Here's the drawing with two shaded views (mm, measured from the low corner). I have some questions. A direction names the side the tool comes from. Coordinates: 2 decimals unless noted, no trailing zeros. Loops run counter-clockwise (first coordinate to the right, second up) from the corner with the lowest first, then second, coordinate; pieces in that order, holes last. Notation, with made-up numbers: (-8.75, 28) - (27.25, 28) arc R32 ccw to (27.25, 55) - close; hole circle Ø9 at (-14, -40). An arc over 180 degrees is marked (long way). One line per item, written item: value. Start each with the question number.
(1) If we mould it in two halves opening along Z, with no side actions, what happens to the marked faces 3, 4 and 5? For each: pulls with the +Z half, pulls with the -Z half, needs draft (parallel to the pull), parting line crosses it, or undercut.
(2) If we section it at A-A on y = 8: Write out the boundary of the cut face in (x, z) (3 decimals), then the cut area to 3 significant figures.
(3) If I drill on line 1 along Z through (x, y) = (2, 8) (3 decimals); line 2 along Z through (x, y) = (5.75, 8) (3 decimals), over which ranges is the centre line in solid material (lowest first)? Write a range as from..to.
(4) I'm going to push flat-ended pins straight in: P1, Ø3, axis at x = 8, y = 13.5, coming from the +Z side; P2, Ø4, axis at x = 5.5, y = 3, coming from the +Z side. Where does each tip first touch, or does it pass through?
(5) If we section it at C-C on x = 9.25: Write out the boundary of the cut face in (y, z) (3 decimals), then the cut area to 3 significant figures.
(6) On a 3-axis mill with a long thin cutter (end or side, diameter ignored), from which of +Z, -Z, +X, -X, +Y, -Y can I reach the whole of each face in a straight line? I mean the marked faces 1 and 2. Say none if no direction works.
(7) If we section it at B-B on x = 6.75: Write out the boundary of the cut face in (y, z) (3 decimals).
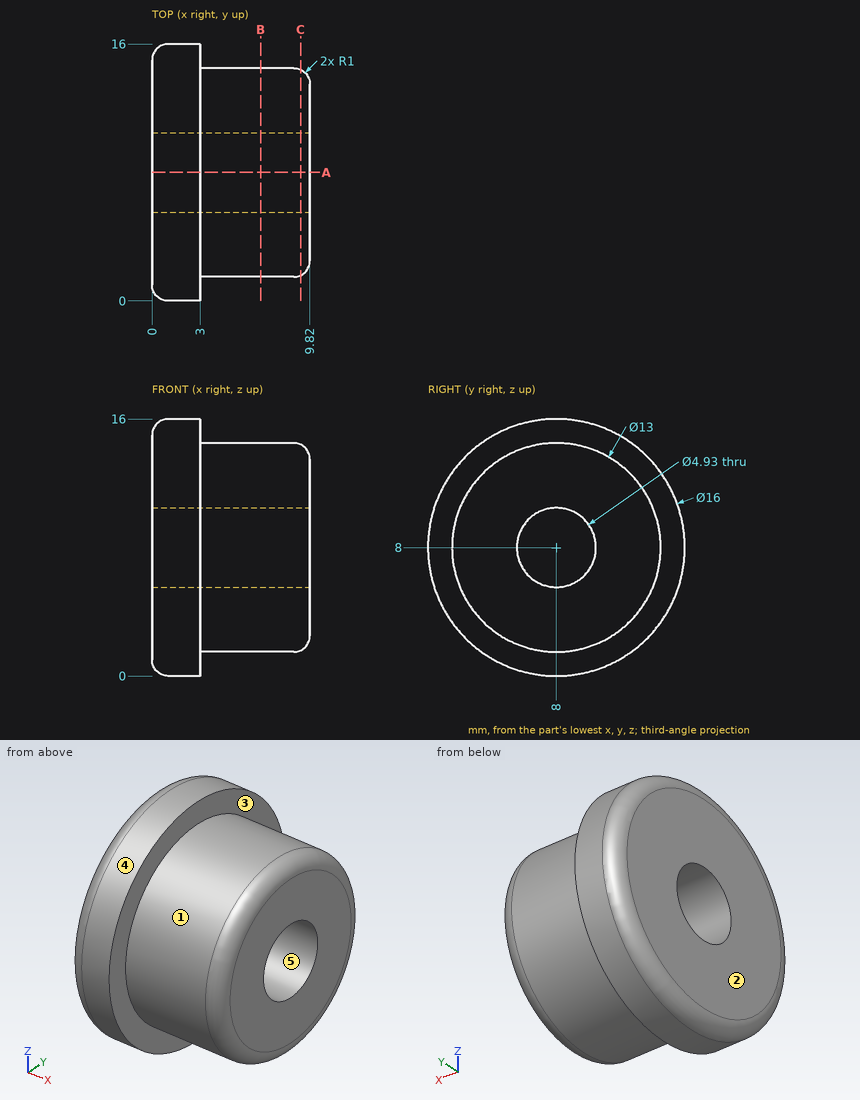
Values:
1. face 3: needs draft
1. face 4: parting line crosses it
1. face 5: undercut
2. outline: (0, 1) arc R1 ccw to (1, 0) - (3, 0) - (3, 1.5) - (8.82, 1.5) arc R1 ccw to (9.82, 2.5) - (9.82, 5.535) - (0, 5.535) - close; (0, 10.465) - (9.82, 10.465) - (9.82, 13.5) arc R1 ccw to (8.82, 14.5) - (3, 14.5) - (3, 16) - (1, 16) arc R1 ccw to (0, 15) - close
2. area: 87.4 mm2
3. line 1: z = 0..5.535, 10.465..16
3. line 2: z = 1.5..5.535, 10.465..14.5
4. P1: stops at z = 13.12
4. P2: stops at z = 13.77
5. outline: circle Ø12.806 at (8, 8); hole circle Ø4.93 at (8, 8)
5. area: 110 mm2
6. face 1: +X
6. face 2: +Z, -Z, -X, +Y, -Y
7. outline: circle Ø13 at (8, 8); hole circle Ø4.93 at (8, 8)
